CAD build for the part. Positions are in the model's coordinates, mm. Round coordinates to 2 decimals unless told otherwise and drop trailing zeros. Write each loop counter-clockwise with the first axis right and the second up, starting at its lowest first coordinate (ties: lowest second). Pieces come first, ordered by that corner, then holes. Notation, with made-up numbers: (51.5, 68) - (59.5, 68) arc R31 ccw to (59.5, 92) - close; hole circle Ø6 at (28.25, 63). An arc over 180 degrees is marked (long way). Put each result on its own line as item: value. Start each with the question number.
Item 1: Cut at B-B (z = 1.75). Count the separate pieces of the cut face and the enclosed holes in it, and give its area (3 significant figures).
Item 2: Cut at D-D (y = 12). Give the cut face in (x, z).
Item 3: Cut at C-C (x = -44.5). Give the cut face in (y, z).
Item 4: Pin check, flat tips, straight feed: pin 1 Ø6 at (x, y) = (25.5, 12) entering from +Z; pin 2 Ø18.5 at (x, y) = (-31.5, 0) entering from -Z; pin 3 Ø3 at (y, z) = (-12.5, 1.5) entering from -X; pin 4 Ø3.5 at (x, y) = (25.5, -5) entering from +Z. Stop position of each tip, or through.
Item 5: Drill centre lines: line 1 (Y direction, x = -31.5, z = 2); line 2 (Y direction, x = 25.5, z = 3.25); line 3 (Y direction, x = -18.5, z = 2.5). Where is each one in solid material? Low to high. Write a range as from..to.
Item 6: Mould opens along X. For faces 1 (the cylindrical face through (-39.492, 0.352, 3.951)), 2 (the cylindrical face through (22.253, -11.857, 3.951)), 3 (the flat face through (-10, 0, 8)), 4 (the flat face through (31.5, 0, 4)) say: released by +X, released by -X, zero draft, split by the parting line, or undercut.
Item 7: Cut at A-A (y = 0). Give the cut face in (x, z), and give its area (4 significant figures).
```python
from build123d import *

# Parameters (mm, degrees)
SKETCH1_R           = 8
SKETCH1_R_2         = 2.25
SKETCH1_R_3         = 3.25
SKETCH1_R_4         = 1.5
BOSS_EXTRUDE1_DEPTH = 8
CHAMFER2_SIZE       = 2
CHAMFER3_SIZE       = 0.5


with BuildPart() as part:
    # Sketch1 → Boss-Extrude1 (new body)
    with BuildSketch(Plane.XY):
        with BuildLine():
            Line((-31.5, -18), (31.5, -18))
            Line((31.5, -18), (31.5, 18))
            Line((31.5, 18), (-31.5, 18))
            ThreePointArc((-31.5, 18), (-49.5, 0), (-31.5, -18))
        make_face()
        with Locations((-31.5, 0)):
            Circle(SKETCH1_R, mode=Mode.SUBTRACT)
        with Locations((-31.5, 13)):
            Circle(SKETCH1_R_2, mode=Mode.SUBTRACT)
        with Locations((-18.5, 0)):
            Circle(SKETCH1_R_2, mode=Mode.SUBTRACT)
        with Locations((-31.5, -13)):
            Circle(SKETCH1_R_2, mode=Mode.SUBTRACT)
        with Locations((-44.5, 0)):
            Circle(SKETCH1_R_2, mode=Mode.SUBTRACT)
        with Locations((25.5, 12)):
            Circle(SKETCH1_R_3, mode=Mode.SUBTRACT)
        with Locations((25.5, 5)):
            Circle(SKETCH1_R_4, mode=Mode.SUBTRACT)
        with Locations((25.5, -5)):
            Circle(SKETCH1_R_4, mode=Mode.SUBTRACT)
        with Locations((25.5, -12)):
            Circle(SKETCH1_R_3, mode=Mode.SUBTRACT)
    extrude(amount=BOSS_EXTRUDE1_DEPTH)

    # Chamfer2
    chamfer2_edges = [part.edges().sort_by_distance(p)[0] for p in [
        (31.5, 18, 4),
        (31.5, -18, 4),
    ]]
    chamfer(chamfer2_edges, length=CHAMFER2_SIZE)

    # Chamfer3
    chamfer3_edges = [part.edges().sort_by_distance(p)[0] for p in [
        (-39.5, 0, 8),
        (22.25, -12, 0),
        (22.25, 12, 0),
        (24, 5, 0),
        (24, -5, 0),
        (-39.5, 0, 0),
        (24, -5, 8),
        (24, 5, 8),
        (22.25, 12, 8),
        (22.25, -12, 8),
    ]]
    chamfer(chamfer3_edges, length=CHAMFER3_SIZE)


solid = part.part
```
Output values:
1. separate pieces: 1
1. enclosed holes: 9
1. area: 2,430 mm2
2. outline: (-44.92, 0) - (-33.52, 0) - (-33.52, 8) - (-44.92, 8) - close; (-29.48, 0) - (21.75, 0) - (22.25, 0.5) - (22.25, 7.5) - (21.75, 8) - (-29.48, 8) - close; (28.75, 0.5) - (29.25, 0) - (31.5, 0) - (31.5, 8) - (29.25, 8) - (28.75, 7.5) - close
3. outline: (-12.45, 0) - (-2.25, 0) - (-2.25, 8) - (-12.45, 8) - close; (2.25, 0) - (12.45, 0) - (12.45, 8) - (2.25, 8) - close
4. pin 1: through
4. pin 2: z = 0
4. pin 3: x = -45.75
4. pin 4: z = 7.75
5. line 1: -18..-15.25, -10.75..-8, 8..10.75, 15.25..18
5. line 2: -18..-15.25, -8.75..-6.5, -3.5..3.5, 6.5..8.75, 15.25..18
5. line 3: -18..-2.25, 2.25..18
6. face 1: undercut
6. face 2: undercut
6. face 3: zero draft
6. face 4: released by +X
7. outline: (-49.5, 0) - (-46.75, 0) - (-46.75, 8) - (-49.5, 8) - close; (-42.25, 0) - (-40, 0) - (-39.5, 0.5) - (-39.5, 7.5) - (-40, 8) - (-42.25, 8) - close; (-23.5, 0.5) - (-23, 0) - (-20.75, 0) - (-20.75, 8) - (-23, 8) - (-23.5, 7.5) - close; (-16.25, 0) - (31.5, 0) - (31.5, 8) - (-16.25, 8) - close
7. area: 447.5 mm2
